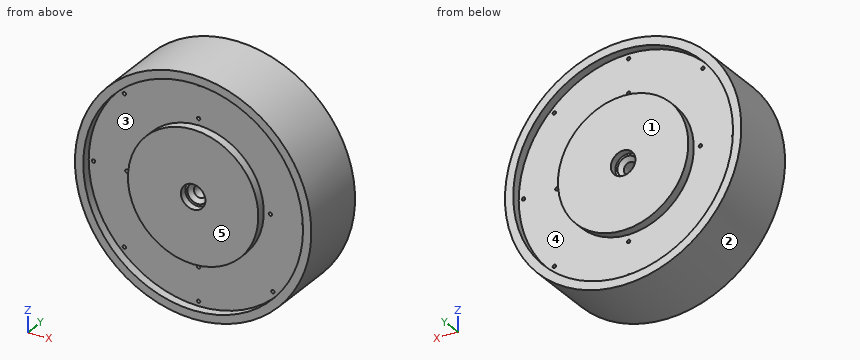
```python
from build123d import *

# Parameters (mm, degrees)
SKETCH1_R           = 135
SKETCH1_R_2         = 7
BOSS_EXTRUDE1_DEPTH = 40
SKETCH2_R           = 14
CUT_EXTRUDE1_DEPTH  = 8
CUT_EXTRUDE2_START  = -72
SKETCH2_3_R         = 14
CUT_EXTRUDE2_DEPTH  = 8
CHAMFER1_SIZE       = 4.5
SKETCH3_W           = 51
SKETCH3_H           = 10
CUT_EXTRUDE3_START  = 30
SKETCH1_3_R         = 1.9
CUT_EXTRUDE3_DEPTH  = 20


with BuildPart() as part:
    # Sketch1 → Boss-Extrude1 (new, symmetric)
    with BuildSketch(Plane(origin=(0, 0, 0), x_dir=(1, 0, 0), z_dir=(0, 1, 0))):
        with Locations(Location((0, 0, 0), (0, 0, 270))):
            Circle(SKETCH1_R)
        with Locations(Location((0, 0, 0), (0, 0, 270))):
            Circle(SKETCH1_R_2, mode=Mode.SUBTRACT)
    extrude(amount=BOSS_EXTRUDE1_DEPTH, both=True)

    # Sketch2 → Cut-Extrude1 (cut)
    with BuildSketch(Plane(origin=(0, 40, 0), x_dir=(1, 0, 0), z_dir=(0, 1, 0))):
        with Locations(Location((0, 0, 0), (0, 0, 270))):
            Circle(SKETCH2_R)
    extrude(amount=-CUT_EXTRUDE1_DEPTH, mode=Mode.SUBTRACT)

    # Sketch2<3> → Cut-Extrude2 (cut)
    with BuildSketch(Plane(origin=(0, 40, 0), x_dir=(1, 0, 0), z_dir=(0, 1, 0)).offset(CUT_EXTRUDE2_START)):
        with Locations(Location((0, 0, 0), (0, 0, 270))):
            Circle(SKETCH2_3_R)
    extrude(amount=-CUT_EXTRUDE2_DEPTH, mode=Mode.SUBTRACT)

    # Chamfer1
    chamfer1_edges = [part.edges().sort_by_distance(p)[0] for p in [
        (0, 32, -7),
        (0, -32, -7),
    ]]
    chamfer(chamfer1_edges, length=CHAMFER1_SIZE)

    # Sketch3 → Cut-Revolve1 (revolve, cut)
    with BuildSketch(Plane(origin=(0, 0, 0), x_dir=(0, 0, -1), z_dir=(1, 0, 0))):
        with Locations((-100, 35)):
            Rectangle(SKETCH3_W, SKETCH3_H)
        with Locations((-100, -35)):
            Rectangle(SKETCH3_W, SKETCH3_H)
    revolve(axis=Axis((0, 58.925226038, 0), (0, -1, 0)), mode=Mode.SUBTRACT)

    # Sketch1<3> → Cut-Extrude3 (cut)
    with BuildSketch(Plane(origin=(0, 0, 0), x_dir=(1, 0, 0), z_dir=(0, 1, 0)).offset(CUT_EXTRUDE3_START)):
        with Locations(Location((0, 120, 0), (0, 0, 90))):
            Circle(SKETCH1_3_R)
        with Locations(Location((84.852813742, 84.852813742, 0), (0, 0, 90))):
            Circle(SKETCH1_3_R)
        with Locations(Location((120, 0, 0), (0, 0, 90))):
            Circle(SKETCH1_3_R)
        with Locations(Location((84.852813742, -84.852813742, 0), (0, 0, 90))):
            Circle(SKETCH1_3_R)
        with Locations(Location((0, -120, 0), (0, 0, 90))):
            Circle(SKETCH1_3_R)
        with Locations(Location((-84.852813742, -84.852813742, 0), (0, 0, 90))):
            Circle(SKETCH1_3_R)
        with Locations(Location((-120, 0, 0), (0, 0, 90))):
            Circle(SKETCH1_3_R)
        with Locations(Location((-84.852813742, 84.852813742, 0), (0, 0, 90))):
            Circle(SKETCH1_3_R)
        with Locations(Location((0, 82, 0), (0, 0, 90))):
            Circle(SKETCH1_3_R)
        with Locations(Location((82, 0, 0), (0, 0, 90))):
            Circle(SKETCH1_3_R)
        with Locations(Location((0, -82, 0), (0, 0, 90))):
            Circle(SKETCH1_3_R)
        with Locations(Location((-82, 0, 0), (0, 0, 90))):
            Circle(SKETCH1_3_R)
    cut_extrude3 = extrude(amount=-CUT_EXTRUDE3_DEPTH, mode=Mode.SUBTRACT)

    # Mirror1: Cut-Extrude3 across plane
    add(cut_extrude3.mirror(Plane.ZX), mode=Mode.SUBTRACT)


solid = part.part
```
Can you work these out from the model? Positions are in its coordinate system, mm. Face numbers are marked on the shaded views. A direction names the side the tool comes from. Round coordinates to 2 decimals unless told otherwise and drop trailing zeros. Loops run counter-clockwise (first coordinate to the right, second up) from the corner with the lowest first, then second, coordinate; pieces in that order, holes last.
Item 1: Please list where these lines run through material, in increasing order: L1, parallel to X at y = 14, z = 0; L2, parallel to Z at x = -35, y = -32; L3, parallel to Y at x = 28, z = -81.5.
Item 2: Suppose I cut it at B-B, the plane z = 43. Write out the boundary of the cut face in (x, y).
Item 3: Suppose I cut it at C-C, the plane x = -99. Write out the boundary of the cut face in (y, z).
Item 4: If we mould it in two halves opening along Z, with no side actions, what happens to the marked faces 1, 2 and 3? For each: +Z half, -Z half, draft (parallel to the pull), parting line (faces both ways), or undercut.
Item 5: Will these pins go through, and if not, where does the flat tip stop? pin 1 Ø1.9 at (x, z) = (84.5, 85.5) entering from +Y; pin 2 Ø3 at (x, z) = (-0.5, 119.5) entering from -Y; pin 3 Ø3 at (x, z) = (-95, -5) entering from +Y.
Item 6: Which directions (+Z, -Z, +X, -X, +Y, -Y) give clear straight access to the entire face, cutting with the end or side of a thin tool? Please do the marked faces 4 and 5.
Item 7: Suppose I cut it at D-D, the plane y = -5.5. Write out the boundary of the cut face in (x, z).
Item 8: Suppose I cut it at A-A, the plane y = 20.5. State how many separate pieces and enclosed holes the cut face has, then the cut area to 3 significant figures.
Reported:
1. L1: x = -135 to -121.9, -118.1 to -83.9, -80.1 to -7, 7 to 80.1, 83.9 to 118.1, 121.9 to 135
1. L2: z = -130.38 to -120.52, -65.77 to 65.77, 120.52 to 130.38
1. L3: y = -30 to 30
2. outline: (-127.97, -40) - (-117.9, -40) - (-117.9, -30) - (-60.84, -30) - (-60.84, -40) - (60.84, -40) - (60.84, -30) - (117.9, -30) - (117.9, -40) - (127.97, -40) - (127.97, 40) - (117.9, 40) - (117.9, 30) - (60.84, 30) - (60.84, 40) - (-60.84, 40) - (-60.84, 30) - (-117.9, 30) - (-117.9, 40) - (-127.97, 40) - close
3. outline: (-40, -91.78) - (40, -91.78) - (40, -77.13) - (30, -77.13) - (30, 77.13) - (40, 77.13) - (40, 91.78) - (-40, 91.78) - (-40, 77.13) - (-30, 77.13) - (-30, -77.13) - (-40, -77.13) - close
4. face 1: draft
4. face 2: parting line
4. face 3: undercut
5. pin 1: stops at y = 10
5. pin 2: stops at y = -30
5. pin 3: stops at y = 30
6. face 4: +Y
6. face 5: +Z, -Z, +X, -X, -Y
7. outline: circle Ø270 at (0, 0); hole circle Ø14 at (0, 0)
8. separate pieces: 1
8. enclosed holes: 13
8. area: 57,000 mm2
